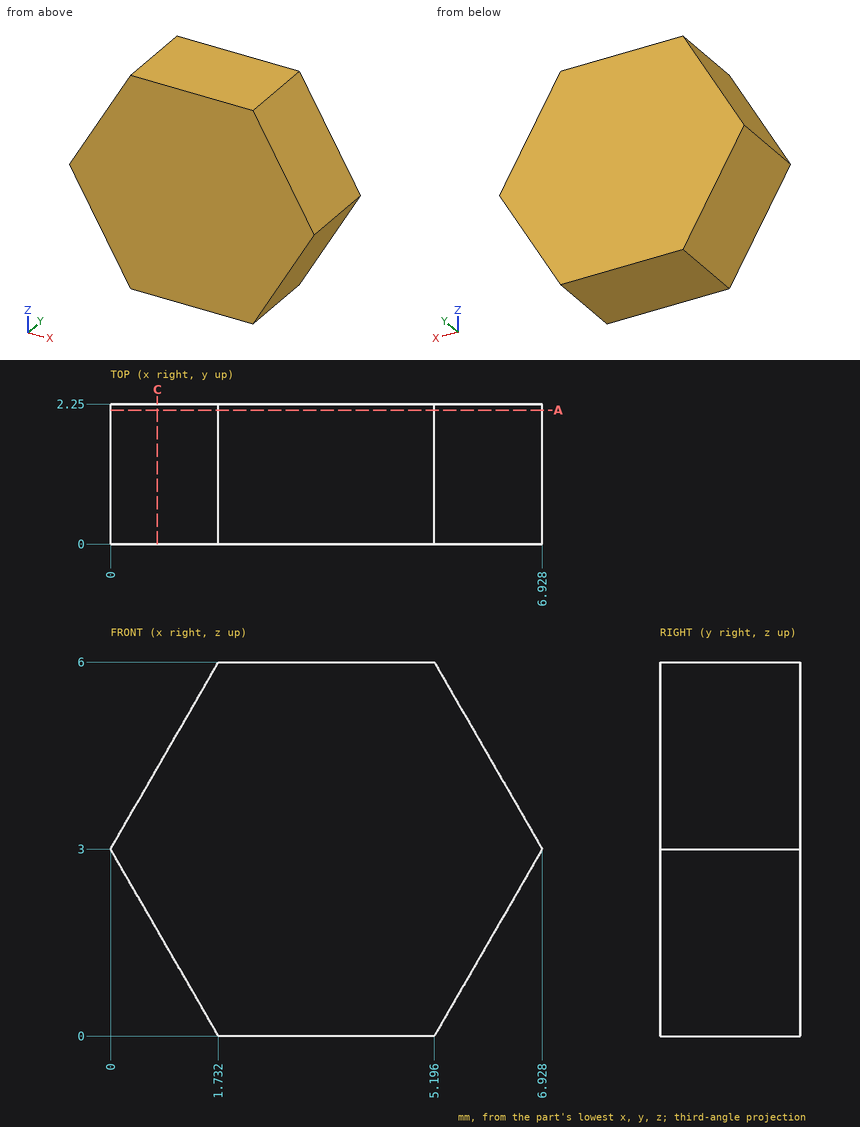
Drawing for the job (mm, zero at the part's lowest x, y, z). Round coordinates to 2 decimals unless told otherwise and drop trailing zeros. Loops run counter-clockwise (first coordinate to the right, second up) from the corner with the lowest first, then second, coordinate; pieces in that order, holes last. Notation, with made-up numbers: M 57.5,37 L 84.5,37 A9 ccw 84.5,52 Z; hole C 64.25,17.25 d5. An arc over 180 degrees is marked long. Use a Markdown table: item, result. Add a question column.
(1) Cut at A-A (y = 2.15). Give the cut face in (x, z).
(2) Drill centre lines: line 1 (X direction, y = 1.25, z = 5.5) (1 decimal); line 2 (X direction, y = 2.2, z = 3.7) (1 decimal); line 3 (Z direction, x = 1, y = 0.7). Where is each one in solid material? Low to high.
(3) Flat gauge pins, fed straight in: pin 1 (1 mm diameter, centred on y = 1.5, z = 5, fed in from +X); pin 2 (1 mm diameter, centred on y = 1, z = 0.5, fed in from -X) (1 decimal). Where does each tip first touch, or does it go through?
(4) Cut at C-C (x = 0.75). Give the cut face in (y, z).
Geometry says:
| question | item | result |
|---|---|---|
| 1 | outline | M 0,3 L 1.73,0 L 5.2,0 L 6.93,3 L 5.2,6 L 1.73,6 Z |
| 2 | line 1 | x = 1.4 to 5.5 |
| 2 | line 2 | x = 0.4 to 6.5 |
| 2 | line 3 | z = 1.27 to 4.73 |
| 3 | pin 1 | stops at x = 6.06 |
| 3 | pin 2 | stops at x = 1.2 |
| 4 | outline | M 0,1.7 L 2.25,1.7 L 2.25,4.3 L 0,4.3 Z |
